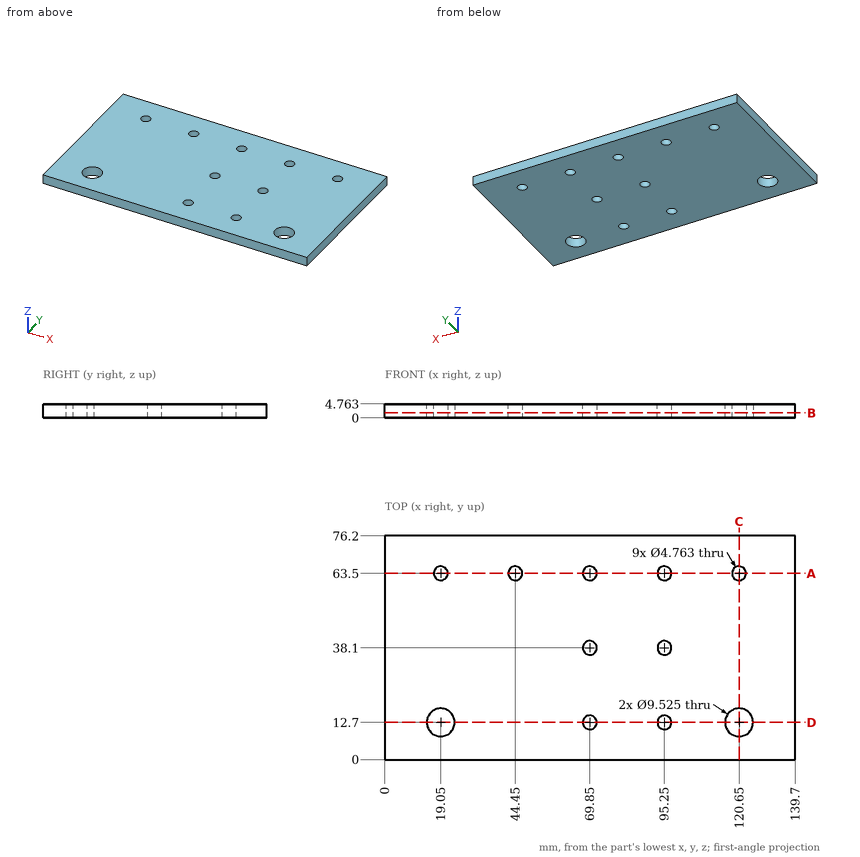
Study the drawing (mm; zero at the part's minimum x, y, z) and answer. Coordinates: 2 decimals unless noted, no trailing zeros. Write each loop counter-clockwise with the first axis right and the second up, starting at its lowest first coordinate (ties: lowest second). Pieces come first, ordered by that corner, then holes. Notation, with made-up numbers: M -18.5,26 L 0.5,26 A24 cw 0.5,46 Z; hole C -11.5,25 d5. An arc over 180 degrees is marked long. Write each question's results on one line, items separated by ' | '.
Item 1: The part is cut by section A-A on y = 63.5. Determine the outline of the cut face in (x, z), and give its area (3 significant figures).
Answer below:
outline: M 0,0 L 16.67,0 L 16.67,4.76 L 0,4.76 Z; M 21.43,0 L 42.07,0 L 42.07,4.76 L 21.43,4.76 Z; M 46.83,0 L 67.47,0 L 67.47,4.76 L 46.83,4.76 Z; M 72.23,0 L 92.87,0 L 92.87,4.76 L 72.23,4.76 Z; M 97.63,0 L 118.27,0 L 118.27,4.76 L 97.63,4.76 Z; M 123.03,0 L 139.7,0 L 139.7,4.76 L 123.03,4.76 Z | area: 552 mm2
Item 2: The part is cut by section B-B on z = 1.75. State how many separate pieces and enclosed holes the cut face has, and give its area (3 significant figures).
Answer below:
separate pieces: 1 | enclosed holes: 11 | area: 10,300 mm2
Item 3: The part is cut by section D-D on y = 12.7. Determine the outline of the cut face in (x, z).
Answer below:
outline: M 0,0 L 14.29,0 L 14.29,4.76 L 0,4.76 Z; M 23.81,0 L 67.47,0 L 67.47,4.76 L 23.81,4.76 Z; M 72.23,0 L 92.87,0 L 92.87,4.76 L 72.23,4.76 Z; M 97.63,0 L 115.89,0 L 115.89,4.76 L 97.63,4.76 Z; M 125.41,0 L 139.7,0 L 139.7,4.76 L 125.41,4.76 Z
Item 4: The part is cut by section C-C on x = 120.65. Determine the outline of the cut face in (y, z).
Answer below:
outline: M 0,0 L 7.94,0 L 7.94,4.76 L 0,4.76 Z; M 17.46,0 L 61.12,0 L 61.12,4.76 L 17.46,4.76 Z; M 65.88,0 L 76.2,0 L 76.2,4.76 L 65.88,4.76 Z
Item 5: Consider probe 1 along Y at (x, z) = (120.65, 2.3); probe 2 along Y at (x, z) = (95.25, 1.2); probe 3 along Y at (x, z) = (44.45, 3.75). Determine where each line is inside the solid, lowest interval first. Write a range as [from, to].
Answer below:
probe 1: [0, 7.94], [17.46, 61.12], [65.88, 76.2] | probe 2: [0, 10.32], [15.08, 35.72], [40.48, 61.12], [65.88, 76.2] | probe 3: [0, 61.12], [65.88, 76.2]
